The model under review builds one solid part; all positions refer to its coordinate system, in mm. Coordinates: 2 decimals unless noted, no trailing zeros. Order: outer loops, then holes, each group sorted by start corner. A loop starts at its lowest first (then second) coordinate and runs counter-clockwise, first axis right, second up.
from build123d import *

# Parameters (mm, degrees)
F0_R      = 19.05
F1_DEPTH  = 1828.8
F2_T      = -2.54
F1_FACE_R = 19.05
F3_DEPTH  = 25.4
F5_W      = 6.35
F5_H      = 30480
F6_DEPTH  = 25.4


with BuildPart() as f1:
    # F0 (on Top) → F1 (new body)
    with BuildSketch(Plane.XY):
        with Locations((-46.609409, 0)):
            Circle(F0_R)
    extrude(amount=F1_DEPTH)

    # F2
    f2_openings = [f1.faces().sort_by_distance(p)[0] for p in [
        (-46.609409, 0, 0),
    ]]
    offset(amount=F2_T, openings=f2_openings)

    # F1_face (on face) → F3 (cut)
    with BuildSketch(Plane(origin=(-46.609409, 0, 1828.8), x_dir=(1, 0, 0), z_dir=(0, 0, 1))):
        Circle(F1_FACE_R)
    extrude(amount=-F3_DEPTH, mode=Mode.SUBTRACT)

    # F5 (on offset) → F6 (cut)
    with BuildSketch(Plane.YZ.offset(-25.4)):
        with Locations((0, 2198.531465)):
            Rectangle(F5_W, F5_H)
    extrude(amount=-F6_DEPTH, mode=Mode.SUBTRACT)


solid = f1.part
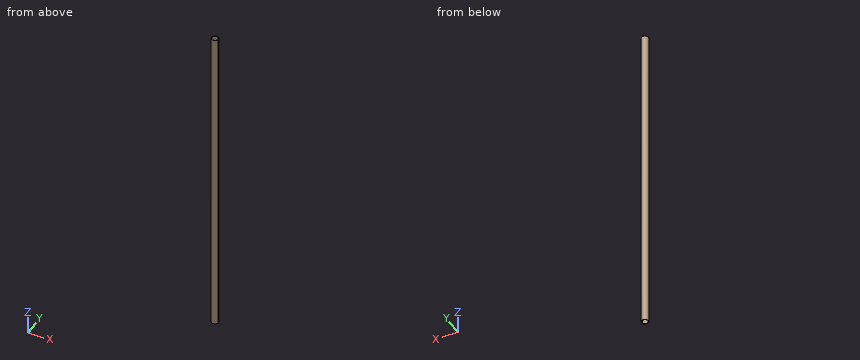
(1) Consider section A-A (x = -56). Give the boundary of the cut face in (y, z), then the cut area to 3 significant figures.
(2) Consider section B-B (z = 396). Give the boundary of the cut face in (x, y) (3 decimals).
(3) Insertion check: pin 1 Ø10 at (x, z) = (-60.5, 1337.5) entering from +Y; pin 2 Ø3 at (x, z) = (-29.5, 1173.5) entering from +Y; pin 3 Ø8 at (x, z) = (-52, 425) entering from -Y; pin 4 Ø6 at (x, y) = (-33, 15) entering from +Z. Each pin has a flat end and moves straight along its axis. Give the tip position at first contact, or say it passes through.
(4) Wall thickness on line 1 (Y direction, x = -46, z = 675); line 2 (X direction, y = 0, z = 960); line 3 (Y direction, x = -33, z = 1243): over which ranges is each line inside the solid? List them lowest first.
Findings:
1. outline: (-16.57, 0) - (-13.58, 0) - (-13.58, 1803.4) - (-16.57, 1803.4) - close; (13.58, 0) - (16.57, 0) - (16.57, 1803.4) - (13.58, 1803.4) - close
1. area: 10,800 mm2
2. outline: (-30.408, -3.175) arc R16.51 cw (long way) to (-30.408, 3.175) - (-27.826, 3.175) arc R19.05 ccw (long way) to (-27.826, -3.175) - close
3. pin 1: stops at y = 16.85
3. pin 2: stops at y = 10.92
3. pin 3: stops at y = -19
3. pin 4: stops at z = 1803.4
4. line 1: y = -19.04 to -16.5, 16.5 to 19.04
4. line 2: x = -65.66 to -63.12
4. line 3: y = -13.33 to -9.35, 9.35 to 13.33
